```python
from build123d import *

# Parameters (mm, degrees)
BOSS_EXTRUDE1_DEPTH = 1.2
SKETCH2_W           = 70
SKETCH2_H           = 435
BOSS_EXTRUDE2_DEPTH = 1.2
BOSS_EXTRUDE3_DEPTH = 1.2
SKETCH4_W           = 52.5
SKETCH4_H           = 70
BOSS_EXTRUDE4_DEPTH = 1.2
CHAMFER1_SIZE       = 30
SKETCH6_W           = 117.5
SKETCH6_H           = 140
BOSS_EXTRUDE5_DEPTH = 1.2


with BuildPart() as part:
    # Sketch1 → Boss-Extrude1 (new body)
    with BuildSketch(Plane(origin=(0, 0, 0), x_dir=(1, 0, 0), z_dir=(0, 1, 0))):
        Polygon((0, 0), (0, 155), (-52.5, 155), (-117.5, 70), (-117.5, 0), align=None)
    extrude(amount=BOSS_EXTRUDE1_DEPTH)

    # Sketch2 → Boss-Extrude2 (add)
    with BuildSketch(Plane.ZY.offset(117.5)):
        with Locations((-35, -216.3)):
            Rectangle(SKETCH2_W, SKETCH2_H)
    extrude(amount=-BOSS_EXTRUDE2_DEPTH)

    # Sketch3 → Boss-Extrude3 (add)
    with BuildSketch(Plane(origin=(-107.920305677, 0, -82.527292576), x_dir=(-0.607450108, 0, 0.794357833), z_dir=(-0.794357833, 0, -0.607450108))):
        Polygon((-91.234333464, 1.2), (15.770339331, 1.2), (15.770339331, -113.122786709), (-91.234333464, -68.8), align=None)
    extrude(amount=-BOSS_EXTRUDE3_DEPTH)

    # Sketch4 → Boss-Extrude4 (add)
    with BuildSketch(Plane(origin=(0, 0, -155), x_dir=(-1, 0, 0), z_dir=(0, 0, -1))):
        with Locations((26.25, -33.8)):
            Rectangle(SKETCH4_W, SKETCH4_H)
    extrude(amount=-BOSS_EXTRUDE4_DEPTH)

    # Chamfer1
    chamfer1_edges = [part.edges().sort_by_distance(p)[0] for p in [
        (-116.9, -433.8, 0),
    ]]
    chamfer(chamfer1_edges, length=CHAMFER1_SIZE)

    # Sketch6 → Boss-Extrude5 (add)
    with BuildSketch(Plane.XY):
        with Locations((-58.75, -68.8)):
            Rectangle(SKETCH6_W, SKETCH6_H)
    extrude(amount=-BOSS_EXTRUDE5_DEPTH)

    # Mirror1: part across face


with BuildPart() as part_1:
    add(part.part)
    add(part.part.mirror(Plane(origin=(0, -32.836293436, -62.654440154), x_dir=(0, 0, 1), z_dir=(1, 0, 0))))


solid = part_1.part
```
For this review, take the finished solid that the model builds, in its own axes (mm). A direction names the side the tool comes from. Round coordinates to 2 decimals unless told otherwise and drop trailing zeros. Write each loop counter-clockwise with the first axis right and the second up, starting at its lowest first coordinate (ties: lowest second). Pieces come first, ordered by that corner, then holes. Notation, with made-up numbers: (33.25, 62) - (75.25, 62) arc R22 ccw to (75.25, 74) - close; hole circle Ø2 at (50, 82). An arc over 180 degrees is marked (long way). Answer as CSV lines item,"result". Start each with the question number.
(1) Add section C-C, the plane z = -47.5. State the section outline as (x, y) points, plus the area to 3 significant figures.
(2) Machinability: for faces 1 (the flat face through (2, -68, -1.2)), 2 (the flat face through (-117.5, -213, -35)), which of the approach directions +Z, -Z, +X, -X, +Y, -Y give a long, thin tool a straight path to every point of the face, cutting with its end or side? Answer none if there is none.
(3) For pin 1 (1 mm diameter, centred on x = 46.5, z = -0.5, fed in from -Y); pin 2 (0.6 mm diameter, centred on x = 7.5, z = -154.5, fed in from -Y); pin 3 (12 mm diameter, centred on x = -16.5, z = -19.5, fed in from -Y), all flat-tipped, find the tip position at first contact; note any pin that passes through.
(4) Add section A-A, the plane y = -248. State the section outline as (x, z) points.
(5) Mouldability with a two-part tool opening along Z and no side actions: class faces 3 (the flat face through (84.377, -43.136, -111.34)), 4 (the flat face through (84.99, -91.27, -111.55)), 5 (the flat face through (-116.3, -214, -35)), 6 (the flat face through (9, -67, 0)) as +Z half, -Z half, draft (parallel to the pull), parting line (faces both ways), or undercut.
(6) Add section B-B, the plane x = 7. State the section outline as (y, z) points, plus the area to 3 significant figures.
(7) For line 1 (X direction, y = -304.5, z = -14.5); line 2 (Y direction, x = -105.5, z = -73.5); line 3 (Z direction, x = 99, y = -57), list the stretches that pass through material, from the lowest coordinate up.
(8) Add section D-D, the plane y = -80.5. State the section outline as (x, z) points.
From the geometry:
1,outline,"(-117.5, -433.8) - (-116.3, -433.8) - (-116.3, 0) - (116.3, 0) - (116.3, -433.8) - (117.5, -433.8) - (117.5, 1.2) - (-117.5, 1.2) - close"
1,area,"1,320 mm²"
2,face 1,"-Y"
2,face 2,"+Z, -Z, -X, +Y, -Y"
3,pin 1,"stops at y = -138.8"
3,pin 2,"stops at y = -68.8"
3,pin 3,"stops at y = 0"
4,outline,"(-117.5, -70) - (-116.3, -70) - (-116.3, 0) - (-117.5, 0) - close; (116.3, -70) - (117.5, -70) - (117.5, 0) - (116.3, 0) - close"
5,face 3,"undercut"
5,face 4,"-Z half"
5,face 5,"undercut"
5,face 6,"+Z half"
6,outline,"(-138.8, -1.2) - (0, -1.2) - (0, -153.8) - (-68.8, -153.8) - (-68.8, -155) - (1.2, -155) - (1.2, 0) - (-138.8, 0) - close"
6,area,"435 mm²"
7,line 1,"x = -117.5 to -116.3, 116.3 to 117.5"
7,line 2,"y = 0 to 1.2"
7,line 3,"z = -94.19 to -92.22, -1.2 to 0"
8,outline,"(-117.5, -70) - (-69.66, -132.56) - (-68.7, -131.83) - (-116.3, -69.59) - (-116.3, -1.2) - (116.3, -1.2) - (116.3, -69.59) - (68.7, -131.83) - (69.66, -132.56) - (117.5, -70) - (117.5, 0) - (-117.5, 0) - close"
